from build123d import *

# Parameters (mm, degrees)
HEXAGONSOCKET_DEPTH = 8


with BuildPart() as part:
    # Sketch1 → Base (revolve)
    with BuildSketch(Plane.XY, mode=Mode.PRIVATE) as base_sk:
        Polygon((0, 0), (20, 0), (20, 7.5), (17.5, 10), (1.353, 10), (0, 8.647), align=None)
    revolve(base_sk.sketch.rotate(Axis((-10.745014543, 0, 0), (1, 0, 0)), 90), axis=Axis((-10.745014543, 0, 0), (1, 0, 0)))

    # Sketch2 → HexagonSocket (cut)
    with BuildSketch(Plane(origin=(0, -0.021932325, 0.010138848), x_dir=(0, 0, 1), z_dir=(-1, 0, 0))):
        Polygon((5.763363844, 0.021932325), (2.876612498, 5.021932325), (-2.896890194, 5.021932325), (-5.78364154, 0.021932325), (-2.896890194, -4.978067675), (2.876612498, -4.978067675), align=None)
    extrude(amount=-HEXAGONSOCKET_DEPTH, mode=Mode.SUBTRACT)

    # Sketch3 → Cut-Revolve1 (revolve, cut)
    with BuildSketch(Plane.XY, mode=Mode.PRIVATE) as cut_revolve1_sk:
        Polygon((8, 5), (10.886751346, 0), (8, 0), align=None)
    revolve(cut_revolve1_sk.sketch.rotate(Axis((-3.144113667, 0, 0), (1, 0, 0)), 90), axis=Axis((-3.144113667, 0, 0), (1, 0, 0)), mode=Mode.SUBTRACT)


solid = part.part
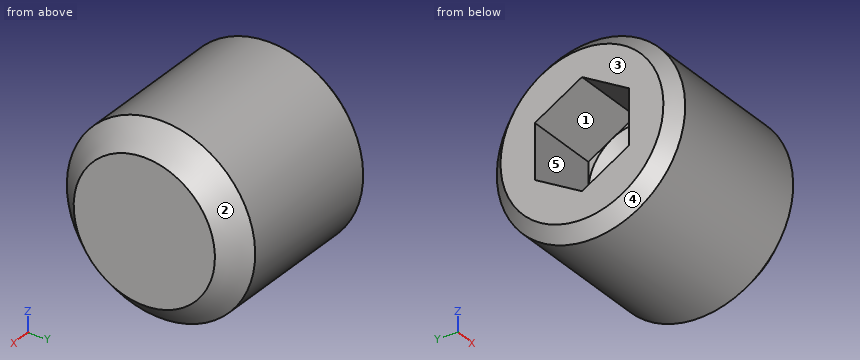
Geometry check sheet. Reference: the model listing, model coordinates, mm. Face numbers are marked on the shaded views. A direction names the side the tool comes from. Round coordinates to 2 decimals unless told otherwise and drop trailing zeros. Write each loop counter-clockwise with the first axis right and the second up, starting at its lowest first coordinate (ties: lowest second). Pieces come first, ordered by that corner, then holes. Notation, with made-up numbers: (-25, -3) -> (-17, -3) arc R23 ccw to (-17, 15) -> close; hole circle Ø11 at (87, 60.25). An arc over 180 degrees is marked (long way). One line per item, written item: value. Start each with the question number.
(1) Cross-section at A-A, the plane x = 9.25. Record the cut outline in (y, z), and give its area (3 significant figures).
(2) Go/stop test with flat-tipped pins: pin 1 Ø8 at (x, z) = (8, 5.5) entering from -Y; pin 2 Ø0.7 at (y, z) = (-3.5, -2) entering from -X; pin 3 Ø2 at (y, z) = (-3.5, 1) entering from -X. Record where each tip stops, or that it passes through.
(3) Access from +Z, -Z, +X, -X, +Y, -Y to the whole of each face (thin tool, end or side, straight path). Record for the marked faces 1 and 2.
(4) Draft check along Z on the marked faces 3, 4 and 5. Enter one of: +Z half, -Z half, draft (parallel to the pull), parting line (faces both ways), or undercut.
(5) Scan lines: line 1 (Y direction, x = 6.25, z = -4.5); line 2 (Z direction, x = 7.75, y = 1.5); line 3 (X direction, y = -1, z = -1). Record each from-to range of solid material in increasing order. Write a range as [from, to].
Answer:
1. outline: circle Ø20 at (0, 0); hole circle Ø5.67 at (0, 0)
1. area: 289 mm²
2. pin 1: y = -9.89
2. pin 2: x = 8.36
2. pin 3: x = 8.21
3. face 1: -X
3. face 2: +X
4. face 3: draft
4. face 4: parting line
4. face 5: undercut
5. line 1: [-8.93, -2.21], [2.21, 8.93]
5. line 2: [-9.89, -4.91], [4.91, 9.89]
5. line 3: [10.07, 20]
